Geometry: final body of the model. Coordinates: model frame, mm. Face numbers are marked on the shaded views. Coordinates: 2 decimals unless noted, no trailing zeros. Order: outer loops, then holes, each group sorted by start corner. A loop starts at its lowest first (then second) coordinate and runs counter-clockwise, first axis right, second up. Notation, with made-up numbers: (-11.5, -6) -> (9.5, -6) arc R20 cw to (9.5, 31) -> close; hole circle Ø4 at (-33.5, -0.75). An arc over 180 degrees is marked (long way). Answer in a Markdown table with one row per item. Add a question column.
1) Pull-direction query (Y, two-part tool) for the marked faces 1, 2, 3 and 4; classes: +Y half, -Y half, draft (parallel to the pull), parting line (faces both ways), or undercut.
2) Section query C-C on y = 8.25. Return the cut outline in (x, z).
3) Section query B-B on x = 18. Return the cut outline in (y, z).
4) Section query A-A on z = 2.75. Return the cut outline in (x, y).
5) Ray query, line 1 (Y direction, x = 18, z = 4.75); line 2 (Z direction, x = -1.5, y = 19.5); line 3 (X direction, y = -33.5, z = 1.5). Return the intervals inside material, ascending. Write a range as from..to.
6) Section query D-D on x = -22.25. Return the cut outline in (y, z), then the cut area to 3 significant figures.
7) Contact query for a flat-ended pin moving along its axis: P1, Ø3, axis at x = 18, y = 8.25, coming from the +Z side. Output: stop coordinate, or through.
```python
from build123d import *

# Parameters (mm, degrees)
SKETCH1_W           = 77.5
SKETCH1_H           = 54.5
BOSS_EXTRUDE1_DEPTH = 2.5
SKETCH1_5_R         = 2.75
SKETCH1_5_R_2       = 1.75
BOSS_EXTRUDE2_DEPTH = 7.5


with BuildPart() as part:
    # Sketch1 → Boss-Extrude1 (new body)
    with BuildSketch(Plane(origin=(0, 0, 0), x_dir=(0, 1, 0), z_dir=(0, 0, 1))):
        Rectangle(SKETCH1_W, SKETCH1_H)
    extrude(amount=-BOSS_EXTRUDE1_DEPTH)

    # Sketch1_5 → Boss-Extrude2 (add)
    # profile 1 of 3: a face of its own
    with BuildSketch(Plane(origin=(0, 0, 0), x_dir=(0, 1, 0), z_dir=(0, 0, 1))):
        with Locations(Location((-33.75, 22.25, 0), (0, 0, 270))):
            Circle(SKETCH1_5_R)
        with Locations(Location((-33.75, 22.25, 0), (0, 0, 270))):
            Circle(SKETCH1_5_R_2, mode=Mode.SUBTRACT)
    # profile 2 of 3: a face of its own
    with BuildSketch(Plane(origin=(0, 0, 0), x_dir=(0, 1, 0), z_dir=(0, 0, 1))):
        with Locations(Location((8.25, -18, 0), (0, 0, 270))):
            Circle(SKETCH1_5_R)
        with Locations(Location((8.25, -18, 0), (0, 0, 270))):
            Circle(SKETCH1_5_R_2, mode=Mode.SUBTRACT)
    # profile 3 of 3: a face of its own
    with BuildSketch(Plane(origin=(0, 0, 0), x_dir=(0, 1, 0), z_dir=(0, 0, 1))):
        with Locations(Location((33.75, 22.25, 0), (0, 0, 270))):
            Circle(SKETCH1_5_R)
        with Locations(Location((33.75, 22.25, 0), (0, 0, 270))):
            Circle(SKETCH1_5_R_2, mode=Mode.SUBTRACT)
    extrude(amount=BOSS_EXTRUDE2_DEPTH)


solid = part.part
```
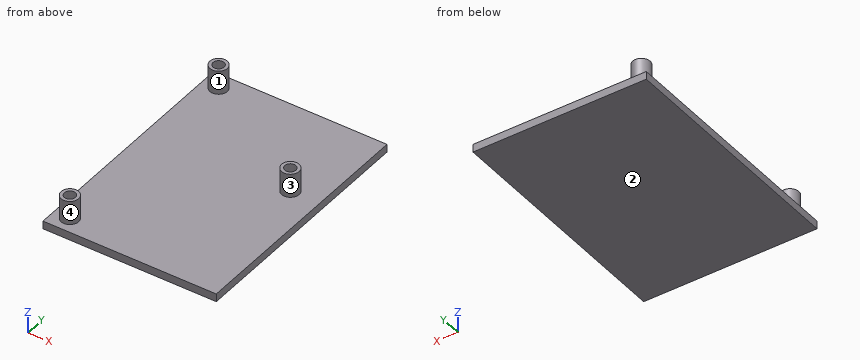
Result:
| question | item | result |
|---|---|---|
| 1 | face 1 | undercut |
| 1 | face 2 | draft |
| 1 | face 3 | parting line |
| 1 | face 4 | undercut |
| 2 | outline | (-27.25, -2.5) -> (27.25, -2.5) -> (27.25, 0) -> (20.75, 0) -> (20.75, 7.5) -> (19.75, 7.5) -> (19.75, 0) -> (16.25, 0) -> (16.25, 7.5) -> (15.25, 7.5) -> (15.25, 0) -> (-27.25, 0) -> close |
| 3 | outline | (-38.75, -2.5) -> (38.75, -2.5) -> (38.75, 0) -> (11, 0) -> (11, 7.5) -> (10, 7.5) -> (10, 0) -> (6.5, 0) -> (6.5, 7.5) -> (5.5, 7.5) -> (5.5, 0) -> (-38.75, 0) -> close |
| 4 | outline | circle Ø5.5 at (-22.25, -33.75); circle Ø5.5 at (-22.25, 33.75); circle Ø5.5 at (18, 8.25); hole circle Ø3.5 at (-22.25, -33.75); hole circle Ø3.5 at (-22.25, 33.75); hole circle Ø3.5 at (18, 8.25) |
| 5 | line 1 | 5.5..6.5, 10..11 |
| 5 | line 2 | -2.5..0 |
| 5 | line 3 | -24.99..-23.98, -20.52..-19.51 |
| 6 | outline | (-38.75, -2.5) -> (38.75, -2.5) -> (38.75, 0) -> (36.5, 0) -> (36.5, 7.5) -> (35.5, 7.5) -> (35.5, 0) -> (32, 0) -> (32, 7.5) -> (31, 7.5) -> (31, 0) -> (-31, 0) -> (-31, 7.5) -> (-32, 7.5) -> (-32, 0) -> (-35.5, 0) -> (-35.5, 7.5) -> (-36.5, 7.5) -> (-36.5, 0) -> (-38.75, 0) -> close |
| 6 | area | 224 mm2 |
| 7 | P1 | z = 0 |
